```python
from build123d import *

# Parameters (mm, degrees)
TABLE_W                      = 99.948937608
TABLE_H                      = 39.897875217
BOSS_EXTRU_1_DEPTH           = 3
PINSPACE_W                   = 7.2
PINSPACE_H                   = 3.2
ENL_V_MAT_EXTRU_1_DEPTH      = 1
ENL_V_MAT_EXTRU_1_DEPTH_BACK = 4
ALCOVE_W                     = 17.4
ALCOVE_H                     = 16.4
ENL_V_MAT_EXTRU_2_DEPTH      = 2
ESQUISSE4_W                  = 0.15303985
ESQUISSE4_H                  = 1.630533914
ESQUISSE4_W_2                = 0.844812891
ESQUISSE4_H_2                = 0.146902924
ENL_V_MAT_EXTRU_3_DEPTH      = 0.5


with BuildPart() as part:
    # table → Boss.-Extru.1 (new body)
    with BuildSketch(Plane.XY):
        with Locations((39.974468804, -9.948937609)):
            Rectangle(TABLE_W, TABLE_H)
    extrude(amount=-BOSS_EXTRU_1_DEPTH)

    # pinspace → Enlèv. mat.-Extru.1 (cut, two sides)
    with BuildSketch(Plane.XY) as enl_v_mat_extru_1_sk:
        with Locations((20, 0)):
            Rectangle(PINSPACE_W, PINSPACE_H)
        Rectangle(PINSPACE_W, PINSPACE_H)
        with Locations((40, 0)):
            Rectangle(PINSPACE_W, PINSPACE_H)
        with Locations((60, 0)):
            Rectangle(PINSPACE_W, PINSPACE_H)
        with Locations((80, 0)):
            Rectangle(PINSPACE_W, PINSPACE_H)
        with Locations((20, -20)):
            Rectangle(PINSPACE_W, PINSPACE_H)
        with Locations((40, -20)):
            Rectangle(PINSPACE_W, PINSPACE_H)
        with Locations((60, -20)):
            Rectangle(PINSPACE_W, PINSPACE_H)
        with Locations((80, -20)):
            Rectangle(PINSPACE_W, PINSPACE_H)
        with Locations((0, -20)):
            Rectangle(PINSPACE_W, PINSPACE_H)
    extrude(amount=ENL_V_MAT_EXTRU_1_DEPTH, mode=Mode.SUBTRACT)
    extrude(enl_v_mat_extru_1_sk.sketch, amount=-ENL_V_MAT_EXTRU_1_DEPTH_BACK, mode=Mode.SUBTRACT)

    # alcove → Enlèv. mat.-Extru.2 (cut)
    with BuildSketch(Plane.XY):
        with Locations((20, 0)):
            Rectangle(ALCOVE_W, ALCOVE_H)
        Rectangle(ALCOVE_W, ALCOVE_H)
        with Locations((40, 0)):
            Rectangle(ALCOVE_W, ALCOVE_H)
        with Locations((60, 0)):
            Rectangle(ALCOVE_W, ALCOVE_H)
        with Locations((80, 0)):
            Rectangle(ALCOVE_W, ALCOVE_H)
        with Locations((20, -20)):
            Rectangle(ALCOVE_W, ALCOVE_H)
        with Locations((40, -20)):
            Rectangle(ALCOVE_W, ALCOVE_H)
        with Locations((60, -20)):
            Rectangle(ALCOVE_W, ALCOVE_H)
        with Locations((80, -20)):
            Rectangle(ALCOVE_W, ALCOVE_H)
        with Locations((0, -20)):
            Rectangle(ALCOVE_W, ALCOVE_H)
    extrude(amount=-ENL_V_MAT_EXTRU_2_DEPTH, mode=Mode.SUBTRACT)

    # Esquisse4 → Enlèv. mat.-Extru.3 (cut)
    with BuildSketch(Plane.XY):
        with Locations((0, 9.355457885)):
            Rectangle(ESQUISSE4_W, ESQUISSE4_H)
        with Locations((20, 9.355457885)):
            Rectangle(ESQUISSE4_W, ESQUISSE4_H)
        with Locations((40, 9.355457885)):
            Rectangle(ESQUISSE4_W, ESQUISSE4_H)
        with Locations((60, 9.355457885)):
            Rectangle(ESQUISSE4_W, ESQUISSE4_H)
        with Locations((80, 9.355457885)):
            Rectangle(ESQUISSE4_W, ESQUISSE4_H)
        with Locations((-9.685415881, 0)):
            Rectangle(ESQUISSE4_W_2, ESQUISSE4_H_2)
        with Locations((-9.685415881, -20)):
            Rectangle(ESQUISSE4_W_2, ESQUISSE4_H_2)
    extrude(amount=-ENL_V_MAT_EXTRU_3_DEPTH, mode=Mode.SUBTRACT)


solid = part.part
```
Input: part model. Units: mm. Frame: model coordinates. A direction names the side the tool comes from. Coordinates: 2 decimals unless noted, no trailing zeros. Write each loop counter-clockwise with the first axis right and the second up, starting at its lowest first coordinate (ties: lowest second). Pieces come first, ordered by that corner, then holes. Notation, with made-up numbers: (37.25, -12) -> (76.25, -12) arc R23 ccw to (76.25, 20) -> close; hole circle Ø11 at (25.5, -12.75). An arc over 180 degrees is marked (long way). Answer as a JSON object with one key per item and string values.
1. Section B-B on y = -3. Return the cut outline in (x, z).
Result set:
{"outline": "(-10, -3) -> (89.95, -3) -> (89.95, 0) -> (88.7, 0) -> (88.7, -2) -> (71.3, -2) -> (71.3, 0) -> (68.7, 0) -> (68.7, -2) -> (51.3, -2) -> (51.3, 0) -> (48.7, 0) -> (48.7, -2) -> (31.3, -2) -> (31.3, 0) -> (28.7, 0) -> (28.7, -2) -> (11.3, -2) -> (11.3, 0) -> (8.7, 0) -> (8.7, -2) -> (-8.7, -2) -> (-8.7, 0) -> (-10, 0) -> close"}
2. Section D-D on z = -1.2. Count the separate pieces of the cut face and the enclosed holes in it, then the cut area to 3 significant figures.
Result set:
{"separate pieces": "1", "enclosed holes": "10", "area": "1,130 mm2"}
3. First-contact query: P1, Ø8, axis at x = 21.5, y = 2, coming from the +Z side. Flat tip, straight axial feed; report the tip coordinate or a pass-through.
Result set:
{"P1": "stops at z = -2"}
4. Section A-A on x = 58. Return the cut outline in (y, z), then the cut area to 3 significant figures.
Result set:
{"outline": "(-29.9, -3) -> (-21.6, -3) -> (-21.6, -2) -> (-28.2, -2) -> (-28.2, 0) -> (-29.9, 0) -> close; (-18.4, -3) -> (-1.6, -3) -> (-1.6, -2) -> (-8.2, -2) -> (-8.2, 0) -> (-11.8, 0) -> (-11.8, -2) -> (-18.4, -2) -> close; (1.6, -3) -> (10, -3) -> (10, 0) -> (8.2, 0) -> (8.2, -2) -> (1.6, -2) -> close", "area": "47.7 mm2"}
5. Access query for faces 4 (the face through (39, -10, -3)), 5 (the face through (80, -22, -2)). Directions: +Z, -Z, +X, -X, +Y, -Y. A direction counts if a zero-diameter tool reaches every point of the face in a straight line with its end or side. Return the directions, or none.
Result set:
{"face 4": "-Z, +X, -X, +Y, -Y", "face 5": "+Z"}
6. Material intervals for line 1 (Y direction, x = -2, z = -0.4); line 2 (X direction, y = -2, z = -1.7); line 3 (X direction, y = 0.5, z = -2.65), sorted ascending. Write a range as from..to.
Result set:
{"line 1": "y = -29.9..-28.2, -11.8..-8.2, 8.2..10", "line 2": "x = -10..-8.7, 8.7..11.3, 28.7..31.3, 48.7..51.3, 68.7..71.3, 88.7..89.95", "line 3": "x = -10..-3.6, 3.6..16.4, 23.6..36.4, 43.6..56.4, 63.6..76.4, 83.6..89.95"}
7. Mould query, pull axis X, two halves, no side actions, for faces 1 (the face through (40, -10, 0)), 2 (the face through (89.949, -10, -1)), 3 (the face through (0, -11.8, -1)). Classes: released by +X, released by -X, zero draft, split by the parting line, or undercut.
Result set:
{"face 1": "zero draft", "face 2": "released by +X", "face 3": "undercut"}
8. Section C-C on x = 35.5. Return the cut outline in (y, z), then the cut area to 3 significant figures.
Result set:
{"outline": "(-29.9, -3) -> (10, -3) -> (10, 0) -> (8.2, 0) -> (8.2, -2) -> (-8.2, -2) -> (-8.2, 0) -> (-11.8, 0) -> (-11.8, -2) -> (-28.2, -2) -> (-28.2, 0) -> (-29.9, 0) -> close", "area": "54.1 mm2"}
